Source: CAD feature listing. Evaluate the final solid. Frame: model axes, mm. Face numbers are marked on the shaded views. A direction names the side the tool comes from. Round coordinates to 2 decimals unless told otherwise and drop trailing zeros. Order: outer loops, then holes, each group sorted by start corner. A loop starts at its lowest first (then second) coordinate and runs counter-clockwise, first axis right, second up. Notation, with made-up numbers: (-35.75, 49.25) -> (-4.75, 49.25) arc R25 ccw to (-4.75, 72.25) -> close; hole circle Ø4 at (68, 55). An arc over 180 degrees is marked (long way). Answer as CSV lines item,"result".
from build123d import *

# Parameters (mm, degrees)
ESQUISSE1_W             = 32
ESQUISSE1_H             = 40
BOSS_EXTRU_1_DEPTH      = 2
ESQUISSE2_W             = 2
ESQUISSE2_H             = 40
BOSS_EXTRU_2_DEPTH      = 28
CONG_1_R                = 20
ESQUISSE3_R             = 4
ENL_V_MAT_EXTRU_1_DEPTH = 30
ESQUISSE4_W             = 10.5
ESQUISSE4_H             = 10.5
ENL_V_MAT_EXTRU_2_DEPTH = 30
ESQUISSE5_W             = 1
ESQUISSE5_H             = 1
ESQUISSE5_W_2           = 10.5
ESQUISSE5_H_2           = 10.5
BOSS_EXTRU_5_DEPTH      = 1.5
ESQUISSE6_W             = 1
ESQUISSE6_H             = 10.5
BOSS_EXTRU_6_DEPTH      = 10.5
ESQUISSE7_R             = 2.5
ENL_V_MAT_EXTRU_3_DEPTH = 10.5
BOSS_EXTRU_7_START      = -16
ESQUISSE8_R             = 4
BOSS_EXTRU_7_DEPTH      = 16


with BuildPart() as part:
    # Esquisse1 → Boss.-Extru.1 (new body)
    with BuildSketch(Plane.XY):
        with Locations((-16, 20)):
            Rectangle(ESQUISSE1_W, ESQUISSE1_H)
    extrude(amount=BOSS_EXTRU_1_DEPTH)

    # Esquisse2 → Boss.-Extru.2 (add)
    with BuildSketch(Plane.XY.offset(2)):
        with Locations((-1, 20)):
            Rectangle(ESQUISSE2_W, ESQUISSE2_H)
    extrude(amount=BOSS_EXTRU_2_DEPTH)

    # Congé1
    cong_1_edges = [part.edges().sort_by_distance(p)[0] for p in [
        (-1, 40, 30),
        (-1, 0, 30),
    ]]
    fillet(cong_1_edges, radius=CONG_1_R - 0.0001)  # a hair under: the kernel refuses the full size

    # Esquisse3 → Enlèv. mat.-Extru.1 (cut)
    with BuildSketch(Plane(origin=(0, 0, 0), x_dir=(0, 0, -1), z_dir=(1, 0, 0))):
        with Locations(Location((-20.5, 20, 0), (0, 0, 90))):
            Circle(ESQUISSE3_R)
    extrude(amount=-ENL_V_MAT_EXTRU_1_DEPTH, mode=Mode.SUBTRACT)

    # Esquisse4 → Enlèv. mat.-Extru.2 (cut)
    with BuildSketch(Plane.XY.offset(2)):
        with Locations((-26.75, 34.75)):
            Rectangle(ESQUISSE4_W, ESQUISSE4_H)
        with Locations((-26.75, 5.25)):
            Rectangle(ESQUISSE4_W, ESQUISSE4_H)
    extrude(amount=-ENL_V_MAT_EXTRU_2_DEPTH, mode=Mode.SUBTRACT)

    # Esquisse5 → Boss.-Extru.5 (add)
    with BuildSketch(Plane.XY.offset(2)):
        with Locations((-21, 29)):
            Rectangle(ESQUISSE5_W, ESQUISSE5_H)
        with Locations((-26.75, 29)):
            Rectangle(ESQUISSE5_W_2, ESQUISSE5_H)
        with Locations((-21, 34.75)):
            Rectangle(ESQUISSE5_W, ESQUISSE5_H_2)
        with Locations((-21, 11)):
            Rectangle(ESQUISSE5_W, ESQUISSE5_H)
        with Locations((-21, 5.25)):
            Rectangle(ESQUISSE5_W, ESQUISSE5_H_2)
        with Locations((-26.75, 11)):
            Rectangle(ESQUISSE5_W_2, ESQUISSE5_H)
    extrude(amount=BOSS_EXTRU_5_DEPTH)

    # Esquisse6 → Boss.-Extru.6 (add)
    with BuildSketch(Plane.ZY.offset(21.5)):
        with Locations((3, 34.75)):
            Rectangle(ESQUISSE6_W, ESQUISSE6_H)
        with Locations((3, 5.25)):
            Rectangle(ESQUISSE6_W, ESQUISSE6_H)
    extrude(amount=BOSS_EXTRU_6_DEPTH)

    # Esquisse7 → Enlèv. mat.-Extru.3 (cut)
    with BuildSketch(Plane.XY.offset(3.5)):
        with Locations((-27, 35)):
            Circle(ESQUISSE7_R)
        with Locations((-27, 5)):
            Circle(ESQUISSE7_R)
    extrude(amount=-ENL_V_MAT_EXTRU_3_DEPTH, mode=Mode.SUBTRACT)

    # Esquisse8 → Boss.-Extru.7 (add)
    with BuildSketch(Plane.ZY.offset(2).offset(BOSS_EXTRU_7_START)):
        with Locations((20.5, 20)):
            Circle(ESQUISSE8_R)
    extrude(amount=BOSS_EXTRU_7_DEPTH)


solid = part.part
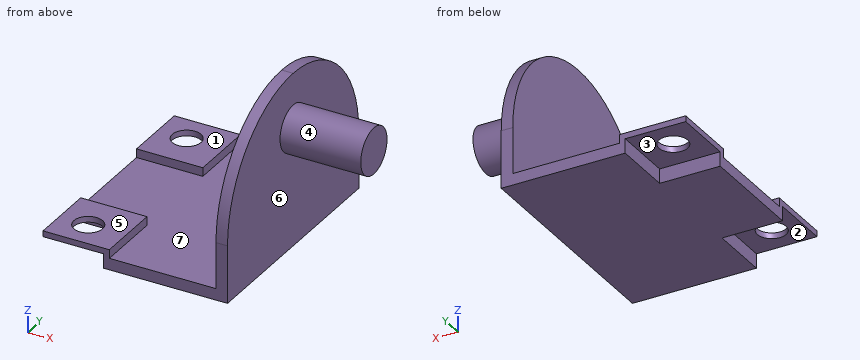
1. Section query B-B on y = 33.5. Return loops of the section in (x, z).
Results below:
outline,"(-32, 2.5) -> (-29, 2.5) -> (-29, 3.5) -> (-32, 3.5) -> close; (-25, 2.5) -> (-21.5, 2.5) -> (-21.5, 0) -> (0, 0) -> (0, 24.76) -> (-2, 24.76) -> (-2, 2) -> (-20.5, 2) -> (-20.5, 3.5) -> (-25, 3.5) -> close"
2. Mould query, pull axis X, two halves, no side actions, for the marked faces 5, 6 and 7. Classes: released by +X, released by -X, zero draft, split by the parting line, or undercut.
Results below:
face 5,"zero draft"
face 6,"released by +X"
face 7,"undercut"
3. Reachability of the marked faces 1, 2, 3 and 4 from +Z, -Z, +X, -X, +Y, -Y: full face, straight path, thin tool, end or side. Return the list, or none.
Results below:
face 1,"+Z, -X, +Y, -Y"
face 2,"-Z, -X, -Y"
face 3,"-Z, -X, +Y"
face 4,"+X"
4. Section query D-D on x = -9. Return loops of the section in (y, z).
Results below:
outline,"(0, 0) -> (40, 0) -> (40, 2) -> (0, 2) -> close"
5. Section query A-A on x = -27. Return loops of the section in (y, z), and give its area (3 significant figures).
Results below:
outline,"(0, 2.5) -> (2.5, 2.5) -> (2.5, 3.5) -> (0, 3.5) -> close; (7.5, 2.5) -> (10.5, 2.5) -> (10.5, 0) -> (29.5, 0) -> (29.5, 2.5) -> (32.5, 2.5) -> (32.5, 3.5) -> (28.5, 3.5) -> (28.5, 2) -> (11.5, 2) -> (11.5, 3.5) -> (7.5, 3.5) -> close; (37.5, 2.5) -> (40, 2.5) -> (40, 3.5) -> (37.5, 3.5) -> close"
area,"52.0 mm2"
6. Section query C-C on z = 20.5. Return loops of the section in (x, y).
Results below:
outline,"(-2, 2.98) -> (0, 2.98) -> (0, 16) -> (14, 16) -> (14, 24) -> (0, 24) -> (0, 37.02) -> (-2, 37.02) -> close"
7. Line query: L1, parallel to Y at x = -27, z = 3; L2, parallel to X at y = 25.5, z = 10.5; L3, parallel to X at y = 22, z = 20.5. Output: solid intervals per line, ascending. Write a range as [from, to].
Results below:
L1,"[0, 2.5], [7.5, 11.5], [28.5, 32.5], [37.5, 40]"
L2,"[-2, 0]"
L3,"[-2, 14]"
8. Pin query (flat end, axial travel): pin 1 (1.2 mm diameter, centred on y = 4, z = 3, fed in from +X); pin 2 (1.2 mm diameter, centred on x = -28, z = 1.5, fed in from +Y); pin 3 (2 mm diameter, centred on y = 17, z = 13, fed in from -X). Return the tip coordinate at first contact, or that it passes through.
Results below:
pin 1,"x = 0"
pin 2,"y = 29.5"
pin 3,"x = -2"
